Can you work these out from the model? Positions are in its coordinate system, mm. Face numbers are marked on the shaded views. A direction names the side the tool comes from. Coordinates: 2 decimals unless noted, no trailing zeros. Order: outer loops, then holes, each group sorted by start corner. A loop starts at its lowest first (then second) coordinate and runs counter-clockwise, first axis right, second up. Notation, with made-up numbers: (71.25, 29.5) -> (90.25, 29.5) arc R10 cw to (90.25, 48.5) -> close; hole circle Ø1 at (25, 81.25). An arc over 180 degrees is marked (long way). Answer in a Markdown table with one row per item. Add a question column.
1. We'd pull the mould along Z, two halves only. Please class the marked faces 3, 4, 5 and 6: pulls with the +Z half, pulls with the -Z half, needs draft (parallel to the pull), parting line crosses it, or undercut.
2. Imagine slicing it at B-B on z = -12.5. Write out the boundary of the cut face in (x, y) (3 decimals), plus the area to 3 significant figures.
3. Imagine slicing it at A-A on x = 0. Write out the boundary of the cut face in (y, z), plus the area to 3 significant figures.
4. Imagine slicing it at D-D on y = 4.75. Write out the boundary of the cut face in (x, z).
5. If I drill on line 1 along X through (y, z) = (0.7, -12.5) (3 decimals); line 2 along X through (y, z) = (4.5, 8.5); line 3 along Y through (x, z) = (-5.5, -7.5), over which ranges is the centre line in solid material (lowest first)? Write a range as [from, to].
6. Imagine slicing it at C-C on z = 8.25. Write out the boundary of the cut face in (x, y), plus the area to 3 significant figures.
7. Will this pin go through, and if not, where does the flat tip stop? pin 1 (8 mm diameter, centred on x = -4, z = -10.5, fed in from +Y).
8. On a 3-axis mill with a long thin cutter (end or side, diameter ignored), from which of +Z, -Z, +X, -X, +Y, -Y can I reach the whole of each face in a straight line? I mean the marked faces 1 and 2. Say none if no direction works.
from build123d import *

# Parameters (mm, degrees)
SKETCH2_W           = 24
SKETCH2_H           = 16.5
SKETCH2_R           = 4
BOSS_EXTRUDE1_DEPTH = 10
SKETCH2_3_W         = 24
SKETCH2_3_H         = 16.5
SKETCH2_3_R         = 1.835
BOSS_EXTRUDE2_DEPTH = 2


with BuildPart() as part:
    # Sketch2 → Boss-Extrude1 (new body)
    with BuildSketch(Plane(origin=(0, 0, 0), x_dir=(1, 0, 0), z_dir=(0, 1, 0))):
        with Locations((0, -8.25)):
            Rectangle(SKETCH2_W, SKETCH2_H)
        with Locations(Location((0, -8.25, 0), (0, 0, 270))):
            Circle(SKETCH2_R, mode=Mode.SUBTRACT)
    extrude(amount=BOSS_EXTRUDE1_DEPTH)

    # Sketch2_3 → Boss-Extrude2 (add)
    with BuildSketch(Plane(origin=(0, 0, 0), x_dir=(1, 0, 0), z_dir=(0, 1, 0))):
        with Locations((0, 8.25)):
            Rectangle(SKETCH2_3_W, SKETCH2_3_H)
        with Locations(Location((-7.95, 12.5, 0), (0, 0, 270))):
            Circle(SKETCH2_3_R, mode=Mode.SUBTRACT)
        with Locations(Location((7.95, 12.5, 0), (0, 0, 270))):
            Circle(SKETCH2_3_R, mode=Mode.SUBTRACT)
    extrude(amount=BOSS_EXTRUDE2_DEPTH)


solid = part.part
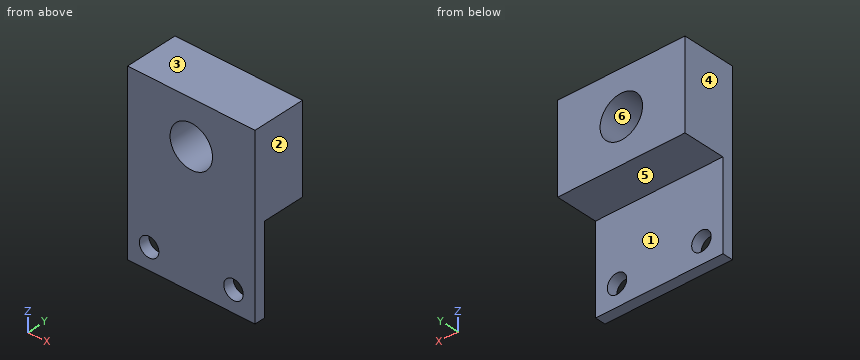
Answers follow:
| question | item | result |
|---|---|---|
| 1 | face 3 | pulls with the +Z half |
| 1 | face 4 | needs draft |
| 1 | face 5 | pulls with the -Z half |
| 1 | face 6 | undercut |
| 2 | outline | (-12, 0) -> (-9.785, 0) -> (-9.785, 2) -> (-12, 2) -> close; (-6.115, 0) -> (6.115, 0) -> (6.115, 2) -> (-6.115, 2) -> close; (9.785, 0) -> (12, 0) -> (12, 2) -> (9.785, 2) -> close |
| 2 | area | 33.3 mm² |
| 3 | outline | (0, -16.5) -> (2, -16.5) -> (2, 0) -> (10, 0) -> (10, 4.25) -> (0, 4.25) -> close; (0, 12.25) -> (10, 12.25) -> (10, 16.5) -> (0, 16.5) -> close |
| 3 | area | 118 mm² |
| 4 | outline | (-12, 0) -> (12, 0) -> (12, 16.5) -> (-12, 16.5) -> close; hole circle Ø8 at (0, 8.25) |
| 5 | line 1 | x = [-12, -9.785], [-6.115, 6.115], [9.785, 12] |
| 5 | line 2 | x = [-12, -3.99], [3.99, 12] |
| 5 | line 3 | y = [0, 2] |
| 6 | outline | (-12, 0) -> (-4, 0) -> (-4, 10) -> (-12, 10) -> close; (4, 0) -> (12, 0) -> (12, 10) -> (4, 10) -> close |
| 6 | area | 160 mm² |
| 7 | pin 1 | stops at y = 2 |
| 8 | face 1 | -Z, +X, -X, +Y |
| 8 | face 2 | +Z, -Z, +X, +Y, -Y |
